The drawing under review shows one solid part. Ordinate dimensions are in mm from its lowest x, y, z. A direction names the side the tool comes from. Coordinates: 2 decimals unless noted, no trailing zeros. Write each loop counter-clockwise with the first axis right and the second up, starting at its lowest first coordinate (ties: lowest second). Pieces come first, ordered by that corner, then holes. Notation, with made-up numbers: (12.5, 26.25) -> (16.5, 26.25) arc R25 ccw to (16.5, 39.25) -> close; hole circle Ø5 at (75.5, -19). An arc over 180 degrees is marked (long way). One line per item, written item: value. Start each with the question number.
1) Add section A-A (z = 30.1). State the section outline as (x, y) points.
2) For probe 1 along X at (y, z) = (1, 34.6); probe 2 along X at (y, z) = (0.85, 30.1); probe 3 along Z at (x, y) = (79.5, 0.6), list the stretches that pass through material, from the lowest coordinate up. Write a range as from..to.
3) Add section D-D (z = 75). State the section outline as (x, y) points, and give its area (3 significant figures).
4) Add section B-B (y = 1.45). State how many separate pieces and enclosed holes the cut face has, and give its area (3 significant figures).
5) Add section C-C (x = 50). State the section outline as (y, z) points.
6) For pin 1 Ø5 at (x, z) = (18.5, 24) entering from +Y; pin 2 Ø2 at (x, z) = (19.5, 121) entering from -Y, all flat-tipped, find the tip position at first contact; note any pin that passes through.
7) Mouldability with a two-part tool opening along X and no side actions: class the marked faces 1 and 2 as released by +X, released by -X, zero draft, split by the parting line, or undercut.
8) Machinability: for the marked faces 3 and 4, which of the approach directions +Z, -Z, +X, -X, +Y, -Y give a long, thin tool a straight path to every point of the face, cutting with its end or side? Answer none if there is none.
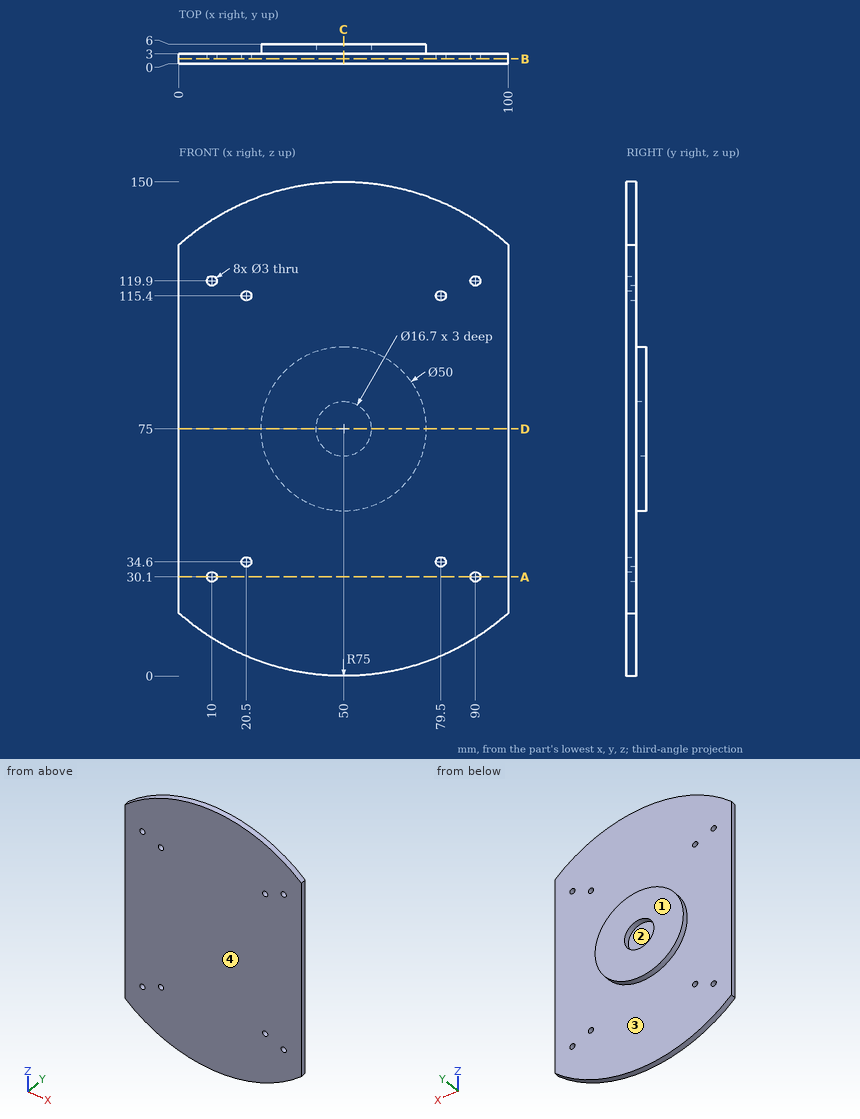
Numbers:
1. outline: (0, 0) -> (8.5, 0) -> (8.5, 3) -> (0, 3) -> close; (11.5, 0) -> (88.5, 0) -> (88.5, 3) -> (11.5, 3) -> close; (91.5, 0) -> (100, 0) -> (100, 3) -> (91.5, 3) -> close
2. probe 1: 0..19, 22..78, 81..100
2. probe 2: 0..8.5, 11.5..88.5, 91.5..100
2. probe 3: 6.05..33.1, 36.1..113.9, 116.9..143.95
3. outline: (0, 0) -> (100, 0) -> (100, 3) -> (75, 3) -> (75, 6) -> (58.35, 6) -> (58.35, 3) -> (41.65, 3) -> (41.65, 6) -> (25, 6) -> (25, 3) -> (0, 3) -> close
3. area: 400 mm²
4. separate pieces: 1
4. enclosed holes: 8
4. area: 13,700 mm²
5. outline: (0, 0) -> (3, 0) -> (3, 50) -> (6, 50) -> (6, 66.65) -> (3, 66.65) -> (3, 83.35) -> (6, 83.35) -> (6, 100) -> (3, 100) -> (3, 150) -> (0, 150) -> close
6. pin 1: y = 3
6. pin 2: y = 0
7. face 1: zero draft
7. face 2: undercut
8. face 3: +Y
8. face 4: +Z, -Z, +X, -X, -Y
